Can you work these out from the model? Positions are in its coordinate system, mm. Round coordinates to 2 decimals unless told otherwise and drop trailing zeros. Loops run counter-clockwise (first coordinate to the right, second up) from the corner with the lowest first, then second, coordinate; pieces in that order, holes last. Notation, with made-up numbers: M 3.25,44.25 L 37.25,44.25 A11 ccw 37.25,51.25 Z; hole C 44,-29 d6. An arc over 180 degrees is marked long. Return JSON: item names as keys, results as strings.
```python
from build123d import *

# Parameters (mm, degrees)
RESSALTO_EXTRUS_O1_DEPTH                       = 19
FILETE2_R                                      = 2
FILETE3_R                                      = 2
FILETE4_R                                      = 2
FURO_ROSCADO_PARA_CONDU_TE_DE_M8X1_252_D       = 8.3
FURO_ROSCADO_PARA_CONDU_TE_DE_M8X1_251_D       = 8.3
FURO_ROSCADO_PARA_CONDU_TE_DE_M8X1_251_DEPTH   = 25
FURO_ROSCADO_PARA_CONDU_TE_DE_M8X1_251_TIP     = 2.493571569
FURO_ROSCADO_PARA_CONDU_TE_DE_M8X1_251_O_D     = 8.3
FURO_ROSCADO_PARA_CONDU_TE_DE_M8X1_251_O_DEPTH = 25
FURO_ROSCADO_PARA_CONDU_TE_DE_M8X1_251_O_TIP   = 2.493571569


with BuildPart() as part:
    # Esboço2 → Ressalto-extrusão1 (new body)
    with BuildSketch(Plane(origin=(0, 0, 0), x_dir=(1, 0, 0), z_dir=(0, 1, 0))):
        with BuildLine():
            Line((-25, -200), (-25, -340))
            Line((-25, -340), (25, -340))
            Line((25, -340), (25, -200))
            ThreePointArc((25, -200), (36.838728685, -156.699788653), (69.061196889, -125.446367362))
            ThreePointArc((69.061196889, -125.446367362), (123.279770024, -72.858344084), (143.2, 0))
            Line((143.2, 0), (143.2, 50))
            Line((143.2, 50), (123.2, 50))
            Line((123.2, 50), (123.2, 0))
            ThreePointArc((123.2, 0), (0, -123.2), (-123.2, 0))
            Line((-123.2, 0), (-123.2, 50))
            Line((-123.2, 50), (-143.2, 50))
            Line((-143.2, 50), (-143.2, 0))
            ThreePointArc((-143.2, 0), (-123.279770024, -72.858344084), (-69.061196889, -125.446367362))
            ThreePointArc((-69.061196889, -125.446367362), (-36.838728685, -156.699788653), (-25, -200))
        make_face()
    extrude(amount=RESSALTO_EXTRUS_O1_DEPTH)

    # Filete2
    filete2_edges = [part.edges().sort_by_distance(p)[0] for p in [
        (-133.2, 19, -50),
        (-133.2, 0, -50),
        (-143.2, 9.5, -50),
        (-123.2, 9.5, -50),
    ]]
    fillet(filete2_edges, radius=FILETE2_R)

    # Filete3
    filete3_edges = [part.edges().sort_by_distance(p)[0] for p in [
        (133.2, 0, -50),
        (123.2, 9.5, -50),
        (143.2, 9.5, -50),
        (133.2, 19, -50),
    ]]
    fillet(filete3_edges, radius=FILETE3_R)

    # Filete4
    filete4_edges = [part.edges().sort_by_distance(p)[0] for p in [
        (0, 0, 340),
        (25, 9.5, 340),
        (-25, 9.5, 340),
        (0, 19, 340),
    ]]
    fillet(filete4_edges, radius=FILETE4_R)

    # Furo roscado para conduíte de M8x1.252 (through all)
    with Locations(Plane(origin=(-12.5, 19, 318), x_dir=(0, 0, 1), z_dir=(0, 1, 0))):
        with Locations((0, 0), (0, 25), (-120, 25), (-120, 0)):
            Hole(FURO_ROSCADO_PARA_CONDU_TE_DE_M8X1_252_D / 2)

    # Furo roscado para conduíte de M8x1.251
    with Locations(Plane(origin=(143.2, 9.5, 0), x_dir=(0, 0, 1), z_dir=(1, 0, 0))):
        with Locations((0, 0)):
            Hole(FURO_ROSCADO_PARA_CONDU_TE_DE_M8X1_251_D / 2, depth=FURO_ROSCADO_PARA_CONDU_TE_DE_M8X1_251_DEPTH)
            with Locations((0, 0, -(FURO_ROSCADO_PARA_CONDU_TE_DE_M8X1_251_DEPTH + FURO_ROSCADO_PARA_CONDU_TE_DE_M8X1_251_TIP / 2))):  # 118° drill point
                Cone(0, FURO_ROSCADO_PARA_CONDU_TE_DE_M8X1_251_D / 2, FURO_ROSCADO_PARA_CONDU_TE_DE_M8X1_251_TIP, mode=Mode.SUBTRACT)

    # Furo roscado para conduíte de M8x1.251 o
    with Locations(Plane(origin=(-143.2, 9.5, 0), x_dir=(0, 0, -1), z_dir=(-1, 0, 0))):
        with Locations((0, 0)):
            Hole(FURO_ROSCADO_PARA_CONDU_TE_DE_M8X1_251_O_D / 2, depth=FURO_ROSCADO_PARA_CONDU_TE_DE_M8X1_251_O_DEPTH)
            with Locations((0, 0, -(FURO_ROSCADO_PARA_CONDU_TE_DE_M8X1_251_O_DEPTH + FURO_ROSCADO_PARA_CONDU_TE_DE_M8X1_251_O_TIP / 2))):  # 118° drill point
                Cone(0, FURO_ROSCADO_PARA_CONDU_TE_DE_M8X1_251_O_D / 2, FURO_ROSCADO_PARA_CONDU_TE_DE_M8X1_251_O_TIP, mode=Mode.SUBTRACT)


solid = part.part
```
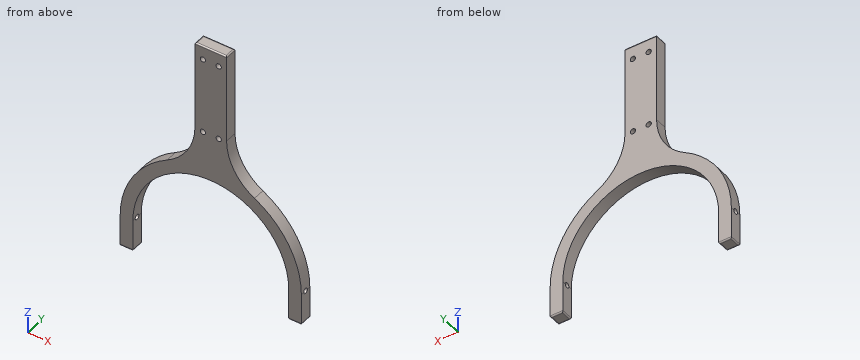
Q1. Suppose I cut it at C-C, the plane x = 12.5. Please give me the cut outline in (y, z), plus the area to 3 significant figures.
Results:
{"outline": "M 0,122.56 L 19,122.56 L 19,193.85 L 0,193.85 Z; M 0,202.15 L 19,202.15 L 19,313.85 L 0,313.85 Z; M 0,322.15 L 19,322.15 L 19,338 A2 ccw 17,340 L 2,340 A2 ccw 0,338 Z", "area": "3,810 mm2"}
Q2. If I drill on line 1 along X through (y, z) = (6.75, 318); line 2 along X through (y, z) = (8.75, -30.5); line 3 along X through (y, z) = (13.75, 62), over which ranges is the centre line in solid material (lowest first)?
Results:
{"line 1": "x = -25 to -16.65, -8.35 to 8.35, 16.65 to 25", "line 2": "x = -143.2 to -123.2, 123.2 to 143.2", "line 3": "x = -129.08 to -106.46, 106.46 to 129.08"}
Q3. Suppose I cut it at A-A, the plane z = 318. Please give me the cut outline in (x, y).
Results:
{"outline": "M -25,0 L -16.65,0 L -16.65,19 L -25,19 Z; M -8.35,0 L 8.35,0 L 8.35,19 L -8.35,19 Z; M 16.65,0 L 25,0 L 25,19 L 16.65,19 Z"}
Q4. I'm going to push flat-ended pins straight in: pin 1 Ø1.5 at (y, z) = (14, 259.5) entering from +X; pin 2 Ø1.5 at (x, y) = (-24, 14.5) entering from -Z; pin 3 Ø8 at (y, z) = (4, 70) entering from -X. Where does each tip first touch, or does it pass through?
Results:
{"pin 1": "stops at x = 25", "pin 2": "stops at z = 120.69", "pin 3": "stops at x = -127.08"}
Q5. Suppose I cut it at B-B, the plane y = 9.5. Please give me the cut outline in (x, z).
Results:
{"outline": "M -143.2,-48 A2 ccw -141.2,-50 L -125.2,-50 A2 ccw -123.2,-48 L -123.2,-4.15 L -143.2,-4.15 Z; M -143.14,4.15 L -123.13,4.15 A123.2 cw 123.13,4.15 L 143.14,4.15 A143.2 ccw 69.06,125.45 A85.1 cw 25,200 L 25,338 A2 ccw 23,340 L -23,340 A2 ccw -25,338 L -25,200 A85.1 cw -69.06,125.45 A143.2 ccw Z; M 123.2,-48 A2 ccw 125.2,-50 L 141.2,-50 A2 ccw 143.2,-48 L 143.2,-4.15 L 123.2,-4.15 Z; hole C -12.5,198 d8.3; hole C -12.5,318 d8.3; hole C 12.5,198 d8.3; hole C 12.5,318 d8.3"}
Q6. Suppose I cut it at D-D, the plane z = 80.5. Please give me the cut outline in (x, y), plus the area to 3 significant figures.
Results:
{"outline": "M -118.43,0 L -93.26,0 L -93.26,19 L -118.43,19 Z; M 93.26,0 L 118.43,0 L 118.43,19 L 93.26,19 Z", "area": "956 mm2"}
